Could you check a few things on this model? Use its own coordinates, in mm. A direction names the side the tool comes from. Round coordinates to 2 decimals unless told otherwise and drop trailing zeros. Write each loop counter-clockwise with the first axis right and the second up, starting at its lowest first coordinate (ties: lowest second). Pieces come first, ordered by that corner, then holes. Notation, with made-up numbers: (51.25, 85.25) - (68.25, 85.25) arc R5 ccw to (68.25, 89.25) - close; hole circle Ø2 at (39, 45). An arc over 180 degrees is marked (long way). Write each question's results on one line, items separated by ' | '. Start each with the question number.
(1) Imagine slicing it at C-C on y = 3.75. Write out the boundary of the cut face in (x, z).
(2) Imagine slicing it at D-D on z = -69.5. Write out the boundary of the cut face in (x, y).
(3) On a 3-axis mill with a long thin cutter (end or side, diameter ignored), from which of +Z, -Z, +X, -X, +Y, -Y can I reach the whole of each face in a straight line? I mean faces 1 (the flat face through (34, 4, -80.5)), 2 (the flat face through (56.576, -1, 9)), 3 (the flat face through (48, -1, -80.2)). Say none if no direction works.
(4) Imagine slicing it at B-B on x = 98.5. Write out the boundary of the cut face in (y, z), then the cut area to 3 significant figures.
(5) For P1, Ø1.9, axis at x = 142.78, z = -86, coming from the +Y side; P2, Ø2.5, axis at x = 142.5, z = -86, coming from the -Y side; P3, Ø2.5, axis at x = 146.5, y = -2, coming from the -Z side, each with a flat end and sliding along its axis, tell me the tip position at first contact or that it passes through.
(6) Imagine slicing it at A-A on z = -3. Write out the boundary of the cut face in (x, y).
(7) Thinking about a two-plate mould opening in X: for faces 4 (the flat face through (98, 2, -47)), 5 (the flat face through (53.788, -1.479, -82.912)), 6 (the flat face through (146, -1, -80.2)), 7 (the flat face through (149.276, -1, -83)), which applies, +X half, -X half, draft (parallel to the pull), parting line (faces both ways), or undercut?
(8) Please list where these lines run through material, in increasing order: line 1 (X direction, y = -0.8, z = 6); line 2 (Z direction, x = 103, y = 2.25); line 3 (Z direction, x = 156.5, y = 4.75). Write a range as [from, to].
```python
from build123d import *

# Parameters (mm, degrees)
SKETCH_1_W      = 129
SKETCH_1_H      = 80
SKETCH_1_R      = 1.6
EXTRUDE_1_DEPTH = 2
SKETCH_2_R      = 2.1
SKETCH_2_W      = 129
SKETCH_2_H      = 80
EXTRUDE_2_DEPTH = 2
EXTRUDE_START   = 3.6
SKETCH_3_R      = 2.1
EXTRUDE_3_DEPTH = 3.6
SKETCH_4_R      = 1.6
EXTRUDE_4_DEPTH = 3


with BuildPart() as part:
    # 草图1 → 凸台-拉伸1 (new body)
    with BuildSketch(Plane(origin=(0, 0, 0), x_dir=(1, 0, 0), z_dir=(0, 1, 0))):
        with Locations((96.776260997, 40)):
            Rectangle(SKETCH_1_W, SKETCH_1_H)
        with Locations(Location((35.276260997, 77, 0), (0, 0, 270))):
            Circle(SKETCH_1_R, mode=Mode.SUBTRACT)
        with Locations(Location((158.276260997, 77, 0), (0, 0, 270))):
            Circle(SKETCH_1_R, mode=Mode.SUBTRACT)
        with Locations(Location((158.276260997, 3, 0), (0, 0, 270))):
            Circle(SKETCH_1_R, mode=Mode.SUBTRACT)
        with Locations(Location((35.276260997, 3, 0), (0, 0, 270))):
            Circle(SKETCH_1_R, mode=Mode.SUBTRACT)
    extrude(amount=EXTRUDE_1_DEPTH)

    # 草图2 → 凸台-拉伸2 (add)
    with BuildSketch(Plane(origin=(0, 2, 0), x_dir=(1, 0, 0), z_dir=(0, 1, 0))):
        with BuildLine():
            Line((35.776260997, 96), (157.776260997, 96))
            ThreePointArc((157.776260997, 96), (162.018901684, 94.242640687), (163.776260997, 90))
            Line((163.776260997, 90), (163.776260997, -10))
            ThreePointArc((163.776260997, -10), (162.018901684, -14.242640687), (157.776260997, -16))
            Line((157.776260997, -16), (35.776260997, -16))
            ThreePointArc((35.776260997, -16), (31.53362031, -14.242640687), (29.776260997, -10))
            Line((29.776260997, -10), (29.776260997, 90))
            ThreePointArc((29.776260997, 90), (31.53362031, 94.242640687), (35.776260997, 96))
        make_face()
        with Locations(Location((35.776260997, -10, 0), (0, 0, 270))):
            Circle(SKETCH_2_R, mode=Mode.SUBTRACT)
        with Locations(Location((157.776260997, -10, 0), (0, 0, 90))):
            Circle(SKETCH_2_R, mode=Mode.SUBTRACT)
        with Locations(Location((157.776260997, 90, 0), (0, 0, 270))):
            Circle(SKETCH_2_R, mode=Mode.SUBTRACT)
        with Locations(Location((35.776260997, 90, 0), (0, 0, 90))):
            Circle(SKETCH_2_R, mode=Mode.SUBTRACT)
        with Locations((96.776260997, 40)):
            Rectangle(SKETCH_2_W, SKETCH_2_H, mode=Mode.SUBTRACT)
    extrude(amount=-EXTRUDE_2_DEPTH)

    # 草图3 → 凸台-拉伸3 (add)
    with BuildSketch(Plane(origin=(0, 2, 0), x_dir=(1, 0, 0), z_dir=(0, 1, 0)).offset(EXTRUDE_START)):
        with BuildLine():
            Line((41.776260997, -10), (41.776260997, -2.5))
            Line((41.776260997, -2.5), (151.776260997, -2.5))
            Line((151.776260997, -2.5), (151.776260997, -10))
            ThreePointArc((151.776260997, -10), (153.53362031, -14.242640687), (157.776260997, -16))
            ThreePointArc((157.776260997, -16), (162.018901684, -14.242640687), (163.776260997, -10))
            Line((163.776260997, -10), (163.776260997, 90))
            ThreePointArc((163.776260997, 90), (162.018901684, 94.242640687), (157.776260997, 96))
            Line((157.776260997, 96), (35.776260997, 96))
            ThreePointArc((35.776260997, 96), (31.53362031, 94.242640687), (29.776260997, 90))
            Line((29.776260997, 90), (29.776260997, -10))
            ThreePointArc((29.776260997, -10), (31.53362031, -14.242640687), (35.776260997, -16))
            ThreePointArc((35.776260997, -16), (40.018901684, -14.242640687), (41.776260997, -10))
        make_face()
        with Locations(Location((35.776260997, -10, 0), (0, 0, 270))):
            Circle(SKETCH_3_R, mode=Mode.SUBTRACT)
        with Locations(Location((35.776260997, 90, 0), (0, 0, 270))):
            Circle(SKETCH_3_R, mode=Mode.SUBTRACT)
        with Locations(Location((157.776260997, 90, 0), (0, 0, 270))):
            Circle(SKETCH_3_R, mode=Mode.SUBTRACT)
        with Locations(Location((157.776260997, -10, 0), (0, 0, 270))):
            Circle(SKETCH_3_R, mode=Mode.SUBTRACT)
        with BuildLine():
            Line((31.776260997, -0.5), (161.776260997, -0.5))
            Line((161.776260997, -0.5), (161.776260997, 80.5))
            Line((161.776260997, 80.5), (157.776260997, 80.5))
            Line((157.776260997, 80.5), (157.776260997, 84))
            ThreePointArc((157.776260997, 84), (152.299035422, 87.550510257), (153.304125042, 94))
            Line((153.304125042, 94), (96.776260997, 94))
            Line((96.776260997, 94), (40.248396952, 94))
            ThreePointArc((40.248396952, 94), (41.253486572, 87.550510257), (35.776260997, 84))
            Line((35.776260997, 84), (35.776260997, 80.5))
            Line((35.776260997, 80.5), (31.776260997, 80.5))
            Line((31.776260997, 80.5), (31.776260997, -0.5))
        make_face(mode=Mode.SUBTRACT)
    extrude(amount=-EXTRUDE_3_DEPTH)

    # 草图4 → 凸台-拉伸4 (add)
    # profile 1 of 4: a face of its own
    with BuildSketch(Plane.XZ):
        with BuildLine():
            Line((149.276260997, -80.2), (142.476260997, -80.2))
            Line((142.476260997, -80.2), (136.976260997, -85.7))
            Line((136.976260997, -85.7), (136.976260997, -92.5))
            Line((136.976260997, -92.5), (142.776260997, -92.5))
            ThreePointArc((142.776260997, -92.5), (147.372455074, -90.596194078), (149.276260997, -86))
            Line((149.276260997, -86), (149.276260997, -80.2))
        make_face()
        with Locations(Location((142.776260997, -86, 0), (0, 0, 270))):
            Circle(SKETCH_4_R, mode=Mode.SUBTRACT)
    # profile 2 of 4: a face of its own
    with BuildSketch(Plane.XZ):
        with BuildLine():
            Line((56.576260997, -92.5), (50.776260997, -92.5))
            ThreePointArc((50.776260997, -92.5), (46.180066919, -90.596194078), (44.276260997, -86))
            Line((44.276260997, -86), (44.276260997, -80.2))
            Line((44.276260997, -80.2), (51.076260997, -80.2))
            Line((51.076260997, -80.2), (56.576260997, -85.7))
            Line((56.576260997, -85.7), (56.576260997, -92.5))
        make_face()
        with Locations(Location((50.776260997, -86, 0), (0, 0, 270))):
            Circle(SKETCH_4_R, mode=Mode.SUBTRACT)
    # profile 3 of 4: a face of its own
    with BuildSketch(Plane.XZ):
        with BuildLine():
            Line((136.976260997, 12.5), (142.776260997, 12.5))
            ThreePointArc((142.776260997, 12.5), (147.372455074, 10.596194078), (149.276260997, 6))
            Line((149.276260997, 6), (149.276260997, 0.2))
            Line((149.276260997, 0.2), (142.476260997, 0.2))
            Line((142.476260997, 0.2), (136.976260997, 5.7))
            Line((136.976260997, 5.7), (136.976260997, 12.5))
        make_face()
        with Locations(Location((142.776260997, 6, 0), (0, 0, 270))):
            Circle(SKETCH_4_R, mode=Mode.SUBTRACT)
    # profile 4 of 4: a face of its own
    with BuildSketch(Plane.XZ):
        with BuildLine():
            Line((44.276260997, 0.2), (51.076260997, 0.2))
            Line((51.076260997, 0.2), (56.576260997, 5.7))
            Line((56.576260997, 5.7), (56.576260997, 12.5))
            Line((56.576260997, 12.5), (50.776260997, 12.5))
            ThreePointArc((50.776260997, 12.5), (46.180066919, 10.596194078), (44.276260997, 6))
            Line((44.276260997, 6), (44.276260997, 0.2))
        make_face()
        with Locations(Location((50.776260997, 6, 0), (0, 0, 270))):
            Circle(SKETCH_4_R, mode=Mode.SUBTRACT)
    extrude(amount=EXTRUDE_4_DEPTH)


solid = part.part
```
Response:
1) outline: (29.78, -90) arc R6 ccw to (35.78, -96) - (157.78, -96) arc R6 ccw to (163.78, -90) - (163.78, 10) arc R6 ccw to (151.78, 10) - (151.78, 2.5) - (41.78, 2.5) - (41.78, 10) arc R6 ccw to (29.78, 10) - close; hole (31.78, -80.5) - (35.78, -80.5) - (35.78, -84) arc R6 cw to (40.25, -94) - (153.3, -94) arc R6 cw to (157.78, -84) - (157.78, -80.5) - (161.78, -80.5) - (161.78, 0.5) - (31.78, 0.5) - close; hole circle Ø4.2 at (35.78, -90); hole circle Ø4.2 at (35.78, 10); hole circle Ø4.2 at (157.78, -90); hole circle Ø4.2 at (157.78, 10)
2) outline: (29.78, 0) - (163.78, 0) - (163.78, 5.6) - (161.78, 5.6) - (161.78, 2) - (31.78, 2) - (31.78, 5.6) - (29.78, 5.6) - close
3) face 1: +Y | face 2: +Z, -Z, -Y | face 3: +X, -X, -Y
4) outline: (0, -96) - (5.6, -96) - (5.6, -94) - (2, -94) - (2, 0.5) - (5.6, 0.5) - (5.6, 2.5) - (2, 2.5) - (2, 16) - (0, 16) - close | area: 238 mm²
5) P1: y = 2 | P2: y = 0 | P3: z = -92.01
6) outline: (29.78, 0) - (33.68, 0) - (33.68, 2) - (31.78, 2) - (31.78, 5.6) - (29.78, 5.6) - close; (36.88, 0) - (156.68, 0) - (156.68, 2) - (36.88, 2) - close; (159.88, 0) - (163.78, 0) - (163.78, 5.6) - (161.78, 5.6) - (161.78, 2) - (159.88, 2) - close
7) face 4: undercut | face 5: undercut | face 6: draft | face 7: +X half
8) line 1: [44.28, 49.18], [52.38, 56.58], [136.98, 141.18], [144.38, 149.28] | line 2: [-96, -94], [0.5, 2.5] | line 3: [-96, -91.67], [-88.33, -84.14], [0.5, 8.33], [11.67, 15.86]
